Build history of the part. All positions in model axes, mm. Face numbers are marked on the shaded views. A direction names the side the tool comes from. Give positions to 0.01 mm unless a question says otherwise; leave off trailing zeros. Loops run counter-clockwise (first coordinate to the right, second up) from the corner with the lowest first, then second, coordinate; pieces in that order, holes last. Notation, with made-up numbers: M -14,-12 L 10,-12 A18 cw 10,7 Z; hole C -3,-40 d8. An arc over 180 degrees is marked long. Put each result on its own line as item: value.
```python
from build123d import *

# Parameters (mm, degrees)
F1_DEPTH = 600
F2_W     = 760
F2_H     = 300
F3_DEPTH = 80
F4_W     = 150
F4_H     = 440
F5_DEPTH = 20
F6_SIZE  = 20
F7_R     = 15


with BuildPart() as f1:
    # F0 (on Front) → F1 (new body)
    with BuildSketch(Plane.XZ):
        Polygon((-220, 0), (0, 0), (0, 290), (-700, 290), (-700, 0), (-480, 0), (-425, 190), (-275, 190), align=None)
    extrude(amount=F1_DEPTH)

    # F2 (on face) → F3 (cut)
    with BuildSketch(Plane(origin=(0, 0, 0), x_dir=(1, 0, 0), z_dir=(0, 0, -1))):
        with Locations((-350, 300)):
            Rectangle(F2_W, F2_H)
    extrude(amount=-F3_DEPTH, mode=Mode.SUBTRACT)

    # F4 (on face) → F5 (cut)
    with BuildSketch(Plane(origin=(0, 0, 190), x_dir=(1, 0, 0), z_dir=(0, 0, -1))):
        with Locations((-350, 300)):
            Rectangle(F4_W, F4_H)
    extrude(amount=-F5_DEPTH, mode=Mode.SUBTRACT)

    # F6
    f6_edges = [f1.edges().sort_by_distance(p)[0] for p in [
        (-700, 0, 145),
        (-700, -300, 290),
        (-350, 0, 290),
        (0, -300, 290),
        (-350, -600, 290),
        (-700, -600, 145),
        (0, -600, 145),
        (0, 0, 145),
    ]]
    chamfer(f6_edges, length=F6_SIZE)

    # F7
    f7_edges = [f1.edges().sort_by_distance(p)[0] for p in [
        (-425, -520, 200),
        (-275, -520, 200),
        (-425, -80, 200),
        (-275, -80, 200),
    ]]
    fillet(f7_edges, radius=F7_R)


solid = f1.part
```
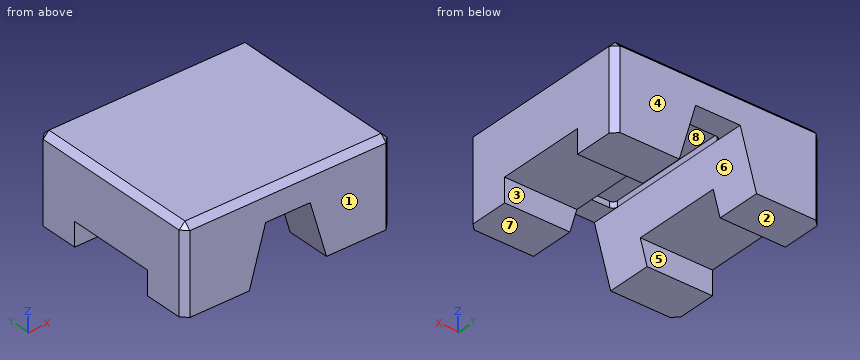
Q1. Drop a flat-ended pin along its axis: pin 1 Ø2 at (x, y) = (-326, -346.5) entering from -Z. Give the stop position or say it passes through.
Here are the results:
pin 1: z = 210
Q2. Slice it at A-A (z = 26). List the corners of the cut face in (x, y).
Here are the results:
outline: M -700,-580 L -680,-600 L -472.47,-600 L -472.47,-450 L -700,-450 Z; M -700,-150 L -472.47,-150 L -472.47,0 L -680,0 L -700,-20 Z; M -227.53,-600 L -20,-600 L 0,-580 L 0,-450 L -227.53,-450 Z; M -227.53,-150 L 0,-150 L 0,-20 L -20,0 L -227.53,0 Z
Q3. Tool access for the marked faces 5, 6, 7 and 8: list every direction of +Z, -Z, +X, -X, +Y, -Y with a clear straight run to the whole face (end or side of a thin tool).
Here are the results:
face 5: -Z, +X, -X
face 6: -Z, +Y, -Y
face 7: -Z, +X, -X, +Y, -Y
face 8: -Z
Q4. Slice it at D-D (x = -379). List the corners of the cut face in (y, z), and give its area (3 significant figures).
Here are the results:
outline: M -600,190 L -520,190 L -520,210 L -80,210 L -80,190 L 0,190 L 0,270 L -20,290 L -580,290 L -600,270 Z
area: 50,800 mm²
Q5. Slice it at C-C (z = 111). List the corners of the cut face in (x, y), and give its area (3 significant figures).
Here are the results:
outline: M -700,-580 L -680,-600 L -447.87,-600 L -447.87,0 L -680,0 L -700,-20 Z; M -252.13,-600 L -20,-600 L 0,-580 L 0,-20 L -20,0 L -252.13,0 Z
area: 302,000 mm²
Q6. Slice it at B-B (y = -128). List the corners of the cut face in (x, z), and give its area (3 significant figures).
Here are the results:
outline: M -700,0 L -480,0 L -425,190 L -425,210 L -275,210 L -275,190 L -220,0 L 0,0 L 0,270 L -20,290 L -680,290 L -700,270 Z
area: 161,000 mm²
Q7. Mould opens along Y. For the marked faces 1, 2, 3 and 4 say: pulls with the +Y half, pulls with the -Y half, needs draft (parallel to the pull), parting line crosses it, or undercut.
Here are the results:
face 1: pulls with the -Y half
face 2: needs draft
face 3: undercut
face 4: pulls with the +Y half
Q8. Probe line 1 (Y direction, x = -484.5, z = 74.5); line 2 (Z direction, x = -43.5, y = -317.5); line 3 (X direction, y = -25, z = 100.5). List the from-to ranges inside material, lowest first. Write a range as from..to.
Here are the results:
line 1: -600..-450, -150..0
line 2: 80..290
line 3: -700..-450.91, -249.09..0
